Could you check a few things on this drawing? It's one solid part, dimensions in mm from its lowest x, y, z. Round coordinates to 2 decimals unless told otherwise and drop trailing zeros. Write each loop counter-clockwise with the first axis right and the second up, starting at its lowest first coordinate (ties: lowest second). Pieces come first, ordered by that corner, then holes. Notation, with made-up numbers: (59, 18) - (86, 18) arc R20 ccw to (86, 33) - close; hole circle Ø4 at (69.5, 76.5). An arc over 180 degrees is marked (long way). One line per question, with ' | ' between items. Start each with the question number.
(1) Imagine slicing it at C-C (x = 37.4). Write out the boundary of the cut face in (y, z).
(2) Thinking about a two-plate mould opening in X: for the marked faces 1, 2 and 3, which applies, pulls with the +X half, pulls with the -X half, needs draft (parallel to the pull), parting line crosses it, or undercut?
(3) If I drill on L1, parallel to X at y = 5.25, z = 29 (1 decimal); L2, parallel to Y at x = 3.5, z = 22.75; L3, parallel to X at y = 1, z = 15, over which ranges is the centre line in solid material (lowest first)?
(4) Will these pins go through, and if not, where does the flat tip stop? pin 1 (3 mm diameter, centred on x = 3.5, y = 4, fed in from -Z); pin 2 (1.5 mm diameter, centred on x = 14.5, y = 4, fed in from -Z) (1 decimal); pin 3 (4 mm diameter, centred on x = 71.3, y = 4, fed in from -Z).
(5) Imagine slicing it at D-D (y = 0.75). Write out the boundary of the cut face in (x, z), plus the area to 3 significant figures.
(6) Imagine slicing it at B-B (y = 4). Give the number of separate pieces and of enclosed holes in the cut face, plus the area to 3 significant figures.
(7) Imagine slicing it at A-A (x = 71.3). Write out the boundary of the cut face in (y, z).
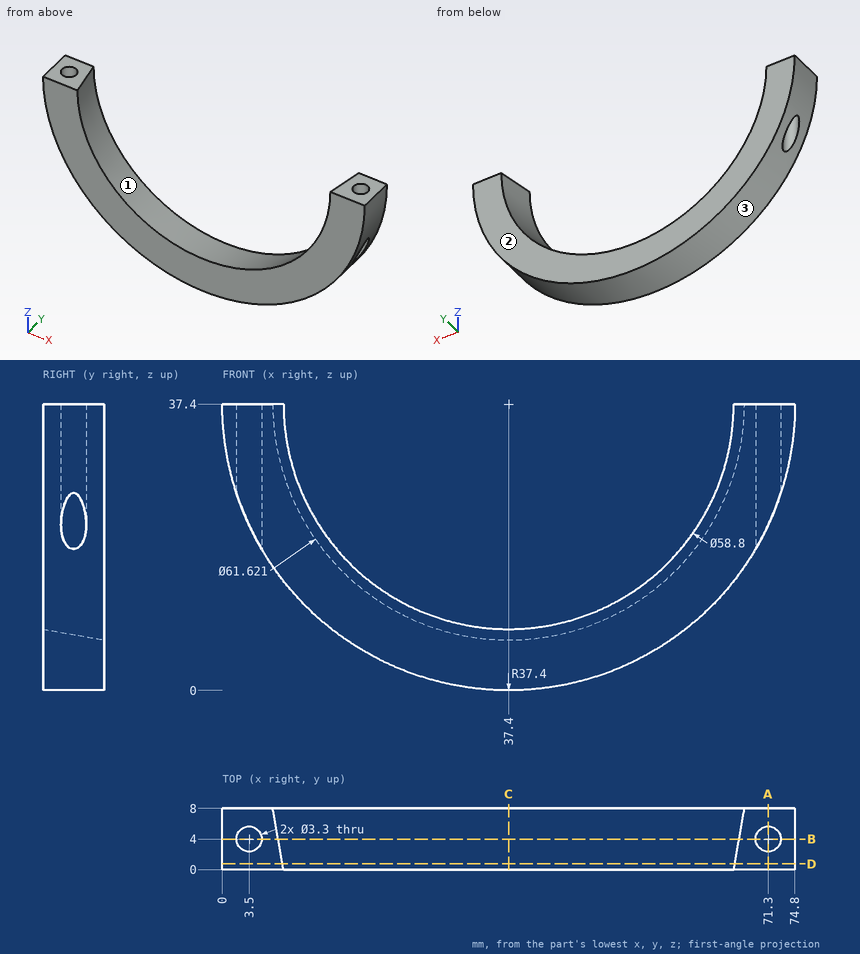
Check sheet entries:
1) outline: (0, 0) - (8, 0) - (8, 6.59) - (0, 8) - close
2) face 1: undercut | face 2: needs draft | face 3: parting line crosses it
3) L1: 1 to 2.4, 4.6 to 8.3, 66.5 to 70.2, 72.4 to 73.8 | L2: 0 to 2.35, 5.65 to 8 | L3: 7.45 to 18.09, 56.71 to 67.35
4) pin 1: through | pin 2: z = 7.3 | pin 3: z = 17.88
5) outline: (0, 37.4) arc R37.4 ccw to (74.8, 37.4) - (66.93, 37.4) arc R29.53 cw to (7.87, 37.4) - close | area: 827 mm^2
6) separate pieces: 3 | enclosed holes: 0 | area: 670 mm^2
7) outline: (0, 21.6) - (2.35, 21.6) - (2.35, 37.4) - (0, 37.4) - close; (5.65, 21.6) - (8, 21.6) - (8, 37.4) - (5.65, 37.4) - close
